```python
from build123d import *

# Parameters (mm, degrees)
F0_R     = 35.0012
F0_R_2   = 29.9974
F1_DEPTH = 15.0114
F0_R_3   = 8.001
F0_R_4   = 9.810431
F2_DEPTH = 15.0114
F0_R_5   = 6.055532
F3_DEPTH = 19.5072


with BuildPart() as f1:
    # F0 (on Front) → F1 (new body)
    with BuildSketch(Plane.XZ):
        Circle(F0_R)
        Circle(F0_R_2, mode=Mode.SUBTRACT)
    extrude(amount=F1_DEPTH)

    # F0 (on Front) → F2 (join)
    with BuildSketch(Plane.XZ):
        Circle(F0_R_2)
        with Locations((0, -19.317703)):
            Circle(F0_R_3, mode=Mode.SUBTRACT)
        with Locations((-20.137208, 0)):
            Circle(F0_R_3, mode=Mode.SUBTRACT)
        Circle(F0_R_4, mode=Mode.SUBTRACT)
        with Locations((21.005314, 0)):
            Circle(F0_R_3, mode=Mode.SUBTRACT)
        with Locations((0, 18.436611)):
            Circle(F0_R_3, mode=Mode.SUBTRACT)
    extrude(amount=F2_DEPTH)

    # F0 (on Front) → F3 (join)
    with BuildSketch(Plane.XZ):
        Circle(F0_R_4)
        Circle(F0_R_5, mode=Mode.SUBTRACT)
    extrude(amount=F3_DEPTH)


solid = f1.part
```
Check sheet for the modelled part. Datum: model origin and axes. Units: mm. A direction names the side the tool comes from. Give positions to 0.01 mm unless a question says otherwise; leave off trailing zeros. Write each loop counter-clockwise with the first axis right and the second up, starting at its lowest first coordinate (ties: lowest second). Pieces come first, ordered by that corner, then holes. Notation, with made-up numbers: (1, 16.5) -> (54, 16.5) arc R15 cw to (54, 39.5) -> close; hole circle Ø8 at (53.25, -38.75). An arc over 180 degrees is marked (long way). Use CSV: the item, a comma, the result in double quotes. Start each with the question number.
Q1. Tool access check on faces 4 (the cylindrical face through (13.01, -7.4, 0.35)), 5 (the flat face through (7.3, -15.011, -7.3)). Record the directions out of +Z, -Z, +X, -X, +Y, -Y that give a thin tool (end or side, any length) a straight path to the whole face; none if there is none.
Q2. Cross-section at D-D on x = 21. Enter the section's corners in (y, z).
Q3. Cross-section at B-B on z = 0. Enter the section's corners in (x, y).
Q4. Depth check by flat-ended pin: P1, Ø4, axis at x = 24.5, z = 23, coming from the -Y side; P2, Ø14, axis at x = 0, z = 0, coming from the -Y side; P3, Ø4, axis at x = 1.5, y = -14.5, coming from the +Z side; P4, Ø14.5, axis at x = 0, z = -19.32, coming from the -Y side. Enter the tip coordinate at first touch or a pass-through.
Q5. Cross-section at C-C on z = -25. Enter the section's corners in (x, y).
Q6. Scan lines: line 1 along Z through (x, y) = (0, -3.75); line 2 along Z through (x, y) = (4.5, -2); line 3 along X through (y, z) = (-3.5, 1). Record each from-to range of solid material in increasing order.
Q7. Cross-section at A-A on x = 0. Enter the section's corners in (y, z).
Q8. Release check for a two-part mould opening along X. For faces 1 (the cylindrical face through (-7.785, -17.228, -5.969)), 2 (the flat face through (-0.1, -19.507, -6.4)), 3 (the cylindrical face through (-1.734, -7.401, 10.626)) record: +X half, -X half, draft (parallel to the pull), parting line (faces both ways), or undercut.
Working result:
1,face 4,"+Y, -Y"
1,face 5,"-Y"
2,outline,"(-15.01, -28) -> (0, -28) -> (0, -8) -> (-15.01, -8) -> close; (-15.01, 8) -> (0, 8) -> (0, 28) -> (-15.01, 28) -> close"
3,outline,"(-35, -15.01) -> (-28.14, -15.01) -> (-28.14, 0) -> (-35, 0) -> close; (-12.14, -15.01) -> (-9.81, -15.01) -> (-9.81, -19.51) -> (-6.06, -19.51) -> (-6.06, 0) -> (-12.14, 0) -> close; (6.06, -19.51) -> (9.81, -19.51) -> (9.81, -15.01) -> (13, -15.01) -> (13, 0) -> (6.06, 0) -> close; (29.01, -15.01) -> (35, -15.01) -> (35, 0) -> (29.01, 0) -> close"
4,P1,"stops at y = -15.01"
4,P2,"stops at y = -19.51"
4,P3,"stops at z = 35"
4,P4,"passes through"
5,outline,"(-24.5, -15.01) -> (-5.63, -15.01) -> (-5.63, 0) -> (-24.5, 0) -> close; (5.63, -15.01) -> (24.5, -15.01) -> (24.5, 0) -> (5.63, 0) -> close"
6,line 1,"z = -35 to -27.32, -11.32 to -6.06, 6.06 to 10.44, 26.44 to 35"
6,line 2,"z = -34.71 to -25.93, -12.7 to -4.05, 4.05 to 11.82, 25.05 to 34.71"
6,line 3,"x = -34.99 to -28.08, -12.2 to -5.97, 5.97 to 13.07, 28.94 to 34.99"
7,outline,"(-19.51, -9.81) -> (-15.01, -9.81) -> (-15.01, -11.32) -> (0, -11.32) -> (0, -6.06) -> (-19.51, -6.06) -> close; (-19.51, 6.06) -> (0, 6.06) -> (0, 10.44) -> (-15.01, 10.44) -> (-15.01, 9.81) -> (-19.51, 9.81) -> close; (-15.01, -35) -> (0, -35) -> (0, -27.32) -> (-15.01, -27.32) -> close; (-15.01, 26.44) -> (0, 26.44) -> (0, 35) -> (-15.01, 35) -> close"
8,face 1,"parting line"
8,face 2,"draft"
8,face 3,"undercut"
